Geometry: final body of the model. Coordinates: model frame, mm. Give positions to 0.01 mm unless a question says otherwise; leave off trailing zeros. Write each loop counter-clockwise with the first axis right and the second up, starting at its lowest first coordinate (ties: lowest second). Pieces come first, ordered by that corner, then holes.
from build123d import *

# Parameters (mm, degrees)
F0_R     = 3.175
F1_DEPTH = 19.05
F2_DEPTH = 22.225
F3_DEPTH = 4.445


# Not quite as in the source:
# - a feature names something its author has since deleted; it is built from what else it names


with BuildPart() as f1:
    # F0 (on Top) → F1 (new body)
    with BuildSketch(Plane.XY):
        with BuildLine():
            ThreePointArc((82.8215071839, 56.5294814298), (0, 37.38), (-82.8215071839, 56.5294814298))
            ThreePointArc((-82.8215071839, 56.5294814298), (-92.8246316261, 54.4975844509), (-93.4439756283, 44.3089870526))
            ThreePointArc((-93.4439756283, 44.3089870526), (-79.88, 0), (-93.4439756283, -44.3089870526))
            ThreePointArc((-93.4439756283, -44.3089870526), (-92.8246316261, -54.4975844509), (-82.8215071839, -56.5294814298))
            ThreePointArc((-82.8215071839, -56.5294814298), (0, -37.38), (82.8215071839, -56.5294814298))
            ThreePointArc((82.8215071839, -56.5294814298), (92.8246316261, -54.4975844509), (93.4439756283, -44.3089870526))
            ThreePointArc((93.4439756283, -44.3089870526), (79.88, 0), (93.4439756283, 44.3089870526))
            ThreePointArc((93.4439756283, 44.3089870526), (92.8246316261, 54.4975844509), (82.8215071839, 56.5294814298))
        make_face()
        with Locations((-55.4007254541, -22.8000469506)):
            Circle(F0_R, mode=Mode.SUBTRACT)
        Circle(F0_R, mode=Mode.SUBTRACT)
        with Locations((55.4007254541, -22.8000469506)):
            Circle(F0_R, mode=Mode.SUBTRACT)
        with Locations((-55.4007254541, 22.8000469506)):
            Circle(F0_R, mode=Mode.SUBTRACT)
        with Locations((55.4007254541, 22.8000469506)):
            Circle(F0_R, mode=Mode.SUBTRACT)
    extrude(amount=F1_DEPTH)

    # F0 (on Top) → F2 (join)
    with BuildSketch(Plane.XY):
        with BuildLine():
            ThreePointArc((82.8215071839, 56.5294814298), (0, 37.38), (-82.8215071839, 56.5294814298))
            ThreePointArc((-82.8215071839, 56.5294814298), (-92.8246316261, 54.4975844509), (-93.4439756283, 44.3089870526))
            ThreePointArc((-93.4439756283, 44.3089870526), (-79.88, 0), (-93.4439756283, -44.3089870526))
            ThreePointArc((-93.4439756283, -44.3089870526), (-92.8246316261, -54.4975844509), (-82.8215071839, -56.5294814298))
            ThreePointArc((-82.8215071839, -56.5294814298), (0, -37.38), (82.8215071839, -56.5294814298))
            ThreePointArc((82.8215071839, -56.5294814298), (92.8246316261, -54.4975844509), (93.4439756283, -44.3089870526))
            ThreePointArc((93.4439756283, -44.3089870526), (79.88, 0), (93.4439756283, 44.3089870526))
            ThreePointArc((93.4439756283, 44.3089870526), (92.8246316261, 54.4975844509), (82.8215071839, 56.5294814298))
        make_face()
        with Locations((-55.4007254541, -22.8000469506)):
            Circle(F0_R, mode=Mode.SUBTRACT)
        Circle(F0_R, mode=Mode.SUBTRACT)
        with Locations((55.4007254541, -22.8000469506)):
            Circle(F0_R, mode=Mode.SUBTRACT)
        with Locations((-55.4007254541, 22.8000469506)):
            Circle(F0_R, mode=Mode.SUBTRACT)
        with Locations((55.4007254541, 22.8000469506)):
            Circle(F0_R, mode=Mode.SUBTRACT)
    extrude(amount=F2_DEPTH)

    # F0 (on Top) → F3 (cut)
    with BuildSketch(Plane.XY):
        with BuildLine():
            ThreePointArc((82.8215071839, 56.5294814298), (0, 37.38), (-82.8215071839, 56.5294814298))
            ThreePointArc((-82.8215071839, 56.5294814298), (-92.8246316261, 54.4975844509), (-93.4439756283, 44.3089870526))
            ThreePointArc((-93.4439756283, 44.3089870526), (-79.88, 0), (-93.4439756283, -44.3089870526))
            ThreePointArc((-93.4439756283, -44.3089870526), (-92.8246316261, -54.4975844509), (-82.8215071839, -56.5294814298))
            ThreePointArc((-82.8215071839, -56.5294814298), (0, -37.38), (82.8215071839, -56.5294814298))
            ThreePointArc((82.8215071839, -56.5294814298), (92.8246316261, -54.4975844509), (93.4439756283, -44.3089870526))
            ThreePointArc((93.4439756283, -44.3089870526), (79.88, 0), (93.4439756283, 44.3089870526))
            ThreePointArc((93.4439756283, 44.3089870526), (92.8246316261, 54.4975844509), (82.8215071839, 56.5294814298))
        make_face()
        with Locations((-55.4007254541, -22.8000469506)):
            Circle(F0_R, mode=Mode.SUBTRACT)
        Circle(F0_R, mode=Mode.SUBTRACT)
        with Locations((55.4007254541, -22.8000469506)):
            Circle(F0_R, mode=Mode.SUBTRACT)
        with Locations((-55.4007254541, 22.8000469506)):
            Circle(F0_R, mode=Mode.SUBTRACT)
        with Locations((55.4007254541, 22.8000469506)):
            Circle(F0_R, mode=Mode.SUBTRACT)
    extrude(amount=F3_DEPTH, mode=Mode.SUBTRACT)


solid = f1.part
Q1. Section B-B on y = 0. Output: boundary loops of the cut face in (x, z) (3 decimals), plus the area to 3 significant figures.
Filled sheet:
outline: (-79.88, 4.445) - (-3.175, 4.445) - (-3.175, 22.225) - (-79.88, 22.225) - close; (3.175, 4.445) - (79.88, 4.445) - (79.88, 22.225) - (3.175, 22.225) - close
area: 2,730 mm2
Q2. Section D-D on z = 16.75. Count the separate pieces of the cut face and the enclosed holes in it, plus the area to 3 significant figures.
Filled sheet:
separate pieces: 1
enclosed holes: 5
area: 15,100 mm2
Q3. Pin query (flat end, axial travel): P1, Ø4, axis at x = -58.5, z = 13.5, coming from the -Y side; P2, Ø10, axis at x = -11, z = 7, coming from the -Y side; P3, Ø1, axis at y = -7, z = 13, coming from the -X side. Return the tip coordinate at first contact, or that it passes through.
Filled sheet:
P1: stops at y = -47.34
P2: stops at y = -38.06
P3: stops at x = -80.24
Q4. Section A-A on x = 0. Output: boundary loops of the cut face in (y, z) (3 decimals).
Filled sheet:
outline: (-37.38, 4.445) - (-3.175, 4.445) - (-3.175, 22.225) - (-37.38, 22.225) - close; (3.175, 4.445) - (37.38, 4.445) - (37.38, 22.225) - (3.175, 22.225) - close
Q5. Ray query, line 1 along X through (y, z) = (-0.5, 17); line 2 along Y through (x, z) = (0, 8.5) (3 decimals); line 3 along X through (y, z) = (25, 7.5). Return the intervals inside material, ascending.
Filled sheet:
line 1: x = -79.88 to -3.14, 3.14 to 79.88
line 2: y = -37.38 to -3.175, 3.175 to 37.38
line 3: x = -83.93 to -57.69, -53.11 to 53.11, 57.69 to 83.93
Q6. Section C-C on x = 55.5. Output: boundary loops of the cut face in (y, z) (1 decimal).
Filled sheet:
outline: (-45.7, 4.4) - (-26, 4.4) - (-26, 22.2) - (-45.7, 22.2) - close; (-19.6, 4.4) - (19.6, 4.4) - (19.6, 22.2) - (-19.6, 22.2) - close; (26, 4.4) - (45.7, 4.4) - (45.7, 22.2) - (26, 22.2) - close
Q7. Pull-direction query (X, two-part tool) for faces 1 (the cylindrical face through (58.33, -24.02, 13.21)), 2 (the cylindrical face through (79.883, -0.658, 13.211)), 3 (the flat face through (-1, -12, 22.225)); classes: released by +X, released by -X, zero draft, split by the parting line, or undercut.
Filled sheet:
face 1: undercut
face 2: released by +X
face 3: zero draft
